CAD build for the part. Positions are in the model's coordinates, mm. Face numbers are marked on the shaded views. A direction names the side the tool comes from. Round coordinates to 2 decimals unless told otherwise and drop trailing zeros. Order: outer loops, then holes, each group sorted by start corner. A loop starts at its lowest first (then second) coordinate and runs counter-clockwise, first axis right, second up. Notation, with made-up numbers: M -28,85.25 L 13,85.25 A27 ccw 13,119.25 Z; hole C 76,78.25 d4. An arc over 180 degrees is marked long. Answer as a JSON object with one key per item and string values. Group by question number.
```python
from build123d import *

# Parameters (mm, degrees)
SKETCH2_R             = 39
SKETCH2_R_2           = 34
BOSS_EXTRUDE1_DEPTH   = 50
SKETCH3_R             = 4
BOSS_EXTRUDE2_DEPTH   = 8
BOSS_EXTRUDE2_2_DEPTH = 8
SKETCH4_R             = 4
BOSS_EXTRUDE3_DEPTH   = 8
BOSS_EXTRUDE3_2_DEPTH = 8
BOSS_EXTRUDE4_START   = -30
BOSS_EXTRUDE4_DEPTH   = 30


with BuildPart() as part:
    # Sketch2 → Boss-Extrude1 (new body)
    with BuildSketch(Plane(origin=(0, 0, 0), x_dir=(1, 0, 0), z_dir=(0, 1, 0))):
        with Locations(Location((0, 0, 0), (0, 0, 270))):
            Circle(SKETCH2_R)
        with Locations(Location((0, 0, 0), (0, 0, 270))):
            Circle(SKETCH2_R_2, mode=Mode.SUBTRACT)
    extrude(amount=BOSS_EXTRUDE1_DEPTH)



with BuildPart() as body_2:
    # Sketch3 → Boss-Extrude2 (new body)
    with BuildSketch(Plane.XY.offset(25.4)):
        with BuildLine():
            Line((-39, 20), (-39, 50))
            Line((-39, 50), (-172.430922253, 97.352057933))
            ThreePointArc((-172.430922253, 97.352057933), (-189.169388202, 90.433792858), (-179.991273047, 74.819669887))
            Line((-179.991273047, 74.819669887), (-39, 20))
        make_face()
        with Locations((-177.792717004, 86.616548767)):
            Circle(SKETCH3_R, mode=Mode.SUBTRACT)
    extrude(amount=-BOSS_EXTRUDE2_DEPTH)


with BuildPart() as body_3:
    # Sketch3 → Boss-Extrude2 2 (new body)
    with BuildSketch(Plane.XY.offset(25.4)):
        with BuildLine():
            Line((39, 50), (39, 20))
            Line((39, 20), (130.917867667, 59.301005864))
            ThreePointArc((130.917867667, 59.301005864), (137.803128547, 75.857402278), (120.557867662, 80.768823316))
            Line((120.557867662, 80.768823316), (39, 50))
        make_face()
        with Locations((126.99576519, 70.641954332)):
            Circle(SKETCH3_R, mode=Mode.SUBTRACT)
    extrude(amount=-BOSS_EXTRUDE2_2_DEPTH)


with BuildPart() as body_4:
    # Sketch4 → Boss-Extrude3 (new body)
    with BuildSketch(Plane.XY.offset(-25.4)):
        with BuildLine():
            Line((39, 50), (120.557867662, 80.768823316))
            ThreePointArc((120.557867662, 80.768823316), (137.803128547, 75.857402278), (130.917867667, 59.301005864))
            Line((130.917867667, 59.301005864), (39, 20))
            Line((39, 20), (39, 50))
        make_face()
        with Locations((126.99576519, 70.641954332)):
            Circle(SKETCH4_R, mode=Mode.SUBTRACT)
    extrude(amount=BOSS_EXTRUDE3_DEPTH)


with BuildPart() as body_5:
    # Sketch4 → Boss-Extrude3 2 (new body)
    with BuildSketch(Plane.XY.offset(-25.4)):
        with BuildLine():
            Line((-172.430922253, 97.352057933), (-39, 50))
            Line((-39, 50), (-39, 20))
            Line((-39, 20), (-179.991273047, 74.819669887))
            ThreePointArc((-179.991273047, 74.819669887), (-189.169388202, 90.433792858), (-172.430922253, 97.352057933))
        make_face()
        with Locations((-177.792717004, 86.616548767)):
            Circle(SKETCH4_R, mode=Mode.SUBTRACT)
    extrude(amount=BOSS_EXTRUDE3_2_DEPTH)


with BuildPart() as part_1:
    add(part.part)

    add(body_2.part)  # Boss-Extrude4 merges body 2

    add(body_3.part)  # Boss-Extrude4 merges body 3

    add(body_4.part)  # Boss-Extrude4 merges body 4

    add(body_5.part)  # Boss-Extrude4 merges body 5
    # Sketch6 → Boss-Extrude4 (add)
    with BuildSketch(Plane(origin=(0, 50, 0), x_dir=(1, 0, 0), z_dir=(0, 1, 0)).offset(BOSS_EXTRUDE4_START)):
        with BuildLine():
            Line((39, 25.4), (39, 17.4))
            Line((39, 17.4), (34.903294973, 17.4))
            ThreePointArc((34.903294973, 17.4), (32.49606782, 21.563987948), (29.594594101, 25.4))
            Line((29.594594101, 25.4), (39, 25.4))
        make_face()
        with BuildLine():
            Line((39, -17.4), (39, -25.4))
            Line((39, -25.4), (29.594594101, -25.4))
            ThreePointArc((29.594594101, -25.4), (32.49606782, -21.563987948), (34.903294973, -17.4))
            Line((34.903294973, -17.4), (39, -17.4))
        make_face()
        with BuildLine():
            Line((-39, -25.4), (-39, -17.4))
            Line((-39, -17.4), (-34.903294973, -17.4))
            ThreePointArc((-34.903294973, -17.4), (-32.49606782, -21.563987948), (-29.594594101, -25.4))
            Line((-29.594594101, -25.4), (-39, -25.4))
        make_face()
        with BuildLine():
            Line((-39, 17.4), (-39, 25.4))
            Line((-39, 25.4), (-29.594594101, 25.4))
            ThreePointArc((-29.594594101, 25.4), (-32.49606782, 21.563987948), (-34.903294973, 17.4))
            Line((-34.903294973, 17.4), (-39, 17.4))
        make_face()
    extrude(amount=BOSS_EXTRUDE4_DEPTH)


solid = part_1.part
```
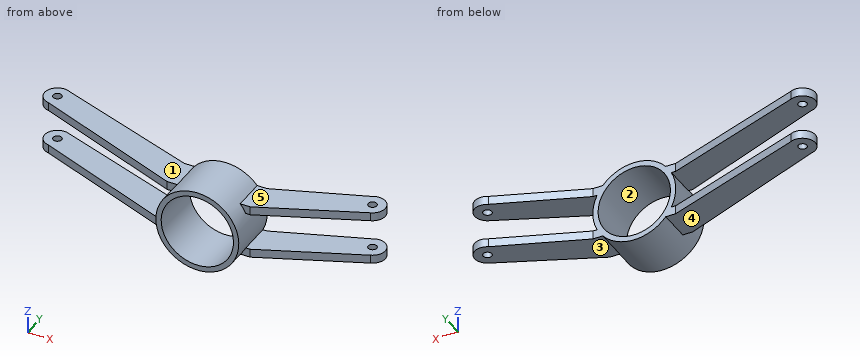
Item 1: Cut at A-A, the plane x = 0. Give the cut face in (y, z), and give its area (3 significant figures).
Item 2: Drill centre lines: line 1 (Z direction, x = 44.5, y = 44); line 2 (Z direction, x = -6, y = 26.5); line 3 (X direction, y = 35, z = 0). Where is each one in solid material? Low to high. Write a range as [from, to].
Item 3: 3-axis set-ups, long thin cutter, end or side, ignore diameter. For the marked faces 4 and 5: which of +Z, -Z, +X, -X, +Y, -Y reach the whole face in a straight line?
Item 4: Cut at C-C, the plane z = 0. Give the cut face in (x, y), and give its area (3 significant figures).
Item 5: Cut at B-B, the plane z = 22. Give the cut face in (x, y), and give its area (3 significant figures).
Item 6: Two-plate mould, pull along Z, no slides. Class the marked faces 1, 2 and 3: +Z half, -Z half, draft (parallel to the pull), parting line (faces both ways), or undercut.
Item 7: Flat gauge pins, fed straight in: pin 1 Ø1.5 at (y, z) = (51.5, -20.5) entering from +X; pin 2 Ø23.5 at (x, y) = (-132.5, 71) entering from +Z; pin 3 Ø1.5 at (y, z) = (46, -14) entering from -X. Where does each tip first touch, or does it go through?
Response values:
{
 "1": {"outline": "M 0,-39 L 50,-39 L 50,-34 L 0,-34 Z; M 0,34 L 50,34 L 50,39 L 0,39 Z", "area": "500 mm^2"},
 "2": {"line 1": "[-25.4, -17.4], [17.4, 25.4]", "line 2": "[-38.54, -33.47], [33.47, 38.54]", "line 3": "[-39, -34], [34, 39]"},
 "3": {"face 4": "-Z, -X, +Y, -Y", "face 5": "+Z, +X, +Y, -Y"},
 "4": {"outline": "M -39,0 L -34,0 L -34,50 L -39,50 Z; M 34,0 L 39,0 L 39,50 L 34,50 Z", "area": "500 mm^2"},
 "5": {"outline": "M -179.99,74.82 L -39,20 L -32.2,20 L -32.2,0 L -25.92,0 L -25.92,50 L -39,50 L -172.43,97.35 A12 ccw long Z; M 25.92,0 L 32.2,0 L 32.2,20 L 39,20 L 130.92,59.3 A12 ccw long 120.56,80.77 L 39,50 L 25.92,50 Z; hole C -177.79,86.62 d8; hole C 127,70.64 d8", "area": "7,670 mm^2"},
 "6": {"face 1": "+Z half", "face 2": "undercut", "face 3": "-Z half"},
 "7": {"pin 1": "x = 114.43", "pin 2": "z = 25.4", "pin 3": "x = -36.68"}
}
